Read the model definition and answer for the solid it produces. Units are mm, in the model's axes. A direction names the side the tool comes from. Give positions to 0.01 mm unless a question says otherwise; leave off trailing zeros. Write each loop counter-clockwise with the first axis right and the second up, starting at its lowest first coordinate (ties: lowest second). Pieces come first, ordered by that corner, then holes. Notation, with made-up numbers: (31, 88.5) -> (83, 88.5) arc R20 ccw to (83, 98.5) -> close; hole circle Ø3 at (19, 26). An arc over 180 degrees is marked (long way). Answer as CSV lines item,"result". Start each with the question number.
1. The part is cut by section A-A, the plane y = 27. Determine the outline of the cut face in (x, z), and give its area (4 significant figures).
2. For a pull along X with two mould halves and no side action, classify faces 1 (the cylindrical face through (0.57, 44.14, 4.45)), 2 (the flat face through (-12, -9, 9)), 3 (the cylindrical face through (6.819, 14.377, 4.437)) as pulls with the +X half, pulls with the -X half, needs draft (parallel to the pull), parting line crosses it, or undercut.
3. The part is cut by section B-B, the plane x = 0. Determine the outline of the cut face in (y, z), and give its area (3 significant figures).
4. Given pin 1 (12 mm diameter, centred on x = -27, y = -10.5, fed in from +Z); pin 2 (5 mm diameter, centred on x = 14, z = 7, fed in from +Y); pin 3 (1 mm diameter, centred on x = 6, z = 5, fed in from -Y), each flat-ended and moving along its own axis, determine where each tip first touches the part or whether it passes through.
5. Find the intervals of material crossed by line 1 (Y direction, x = -14.5, z = 2.75); line 2 (X direction, y = -23, z = 5.25); line 3 (Y direction, x = -1, z = 2.75), in increasing order.
6. A tool of negligible diameter and unlimited length cuts with its end or side. For faces 4 (the cylindrical face through (-8.82, -13.48, 4.44)), 5 (the cylindrical face through (-32.866, -20.771, 5.198)), from which of +Z, -Z, +X, -X, +Y, -Y can it reach the whole face along a straight path? Write none if from no direction.
7. The part is cut by section C-C, the plane z = 2.5. Give the number of separate pieces and of enclosed holes in the cut face, and give its area (3 significant figures).
from build123d import *

# Parameters (mm, degrees)
F0_R     = 11.95
F0_R_2   = 1.705642275
F0_R_3   = 11
F1_DEPTH = 9
F2_SIZE  = 1
F0_R_4   = 10
F3_DEPTH = 1.5


# Not quite as in the source:
# - a fillet or chamfer that OpenCascade refuses, or shapes differently, is made with other operations: its cross-section is extruded or revolved along the edge and cut away or added


with BuildPart() as f1:
    # F0 (on Top) → F1 (new body)
    with BuildSketch(Plane.XY):
        with BuildLine():
            ThreePointArc((18.9439392787, 3.0656279209), (11.0053071194, 6.3539170279), (12.1268812973, 14.8731187027))
            ThreePointArc((12.1268812973, 14.8731187027), (0, 44.15), (-12.1268812973, 14.8731187027))
            ThreePointArc((-12.1268812973, 14.8731187027), (-11.0053071194, 6.3539170279), (-18.9439392787, 3.0656279209))
            ThreePointArc((-18.9439392787, 3.0656279209), (-38.2350215771, -22.075), (-6.8170579813, -17.9387466235))
            ThreePointArc((-6.8170579813, -17.9387466235), (0, -12.7078340558), (6.8170579813, -17.9387466235))
            ThreePointArc((6.8170579813, -17.9387466235), (38.2350215771, -22.075), (18.9439392787, 3.0656279209))
        make_face()
        with Locations((-23.3826859022, -13.5)):
            Circle(F0_R, mode=Mode.SUBTRACT)
        with Locations((-7.4659583891, -12.4409667216)):
            Circle(F0_R_2, mode=Mode.SUBTRACT)
        with Locations((-14.5071724231, -0.2452262678)):
            Circle(F0_R_2, mode=Mode.SUBTRACT)
        with Locations((7.4659583891, -12.4409667216)):
            Circle(F0_R_2, mode=Mode.SUBTRACT)
        with Locations((23.3826859022, -13.5)):
            Circle(F0_R, mode=Mode.SUBTRACT)
        Circle(F0_R_3, mode=Mode.SUBTRACT)
        with Locations((14.5071724231, -0.2452262678)):
            Circle(F0_R_2, mode=Mode.SUBTRACT)
        with Locations((-7.041214034, 12.6861929893)):
            Circle(F0_R_2, mode=Mode.SUBTRACT)
        with Locations((7.041214034, 12.6861929893)):
            Circle(F0_R_2, mode=Mode.SUBTRACT)
        with Locations((0, 27)):
            Circle(F0_R, mode=Mode.SUBTRACT)
    extrude(amount=F1_DEPTH)

    # F2
    f2_edges = [f1.edges().sort_by_distance(p)[0] for p in [
        (-38.235022, -22.075, 9),
        (0, -12.707834, 9),
        (38.235022, -22.075, 9),
        (38.235022, -22.075, 0),
        (0, -12.707834, 0),
        (-38.235022, -22.075, 0),
        (-11.005307, 6.353917, 9),
        (-11.005307, 6.353917, 0),
        (0, 44.15, 0),
        (0, 44.15, 9),
        (11.005307, 6.353917, 9),
        (11.005307, 6.353917, 0),
    ]]
    chamfer(f2_edges, length=F2_SIZE)

    # F0 (on Top) → F3 (join)
    with BuildSketch(Plane.XY):
        with Locations((0, 27)):
            Circle(F0_R)
        with Locations((0, 27)):
            Circle(F0_R_4, mode=Mode.SUBTRACT)
        with Locations((-23.3826859022, -13.5)):
            Circle(F0_R)
        with Locations((-23.3826859022, -13.5)):
            Circle(F0_R_4, mode=Mode.SUBTRACT)
        with Locations((23.3826859022, -13.5)):
            Circle(F0_R)
        with Locations((23.3826859022, -13.5)):
            Circle(F0_R_4, mode=Mode.SUBTRACT)
    extrude(amount=F3_DEPTH)

    # F4: chamfer of 1 on 1 edges, made by hand

    # F4_s1 → F4_t2 (revolve, cut)
    with BuildSketch(Plane.XZ):
        Polygon((12, 9), (11, 8), (11, 9), align=None)
    revolve(axis=Axis((0, 0, 9), (0, 0, 1)), mode=Mode.SUBTRACT)


solid = f1.part
Results found:
1,outline,"(-17.15, 1) -> (-16.15, 0) -> (-10, 0) -> (-10, 1.5) -> (-11.95, 1.5) -> (-11.95, 9) -> (-16.15, 9) -> (-17.15, 8) -> close; (10, 0) -> (16.15, 0) -> (17.15, 1) -> (17.15, 8) -> (16.15, 9) -> (11.95, 9) -> (11.95, 1.5) -> (10, 1.5) -> close"
1,area,"97.45 mm²"
2,face 1,"parting line crosses it"
2,face 2,"needs draft"
2,face 3,"undercut"
3,outline,"(-12.71, 1) -> (-11.71, 0) -> (-11, 0) -> (-11, 8) -> (-11.85, 8.85) -> (-12.71, 8) -> close; (11, 0) -> (17, 0) -> (17, 1.5) -> (15.05, 1.5) -> (15.05, 9) -> (12, 9) -> (11, 8) -> close; (37, 0) -> (43.15, 0) -> (44.15, 1) -> (44.15, 8) -> (43.15, 9) -> (38.95, 9) -> (38.95, 1.5) -> (37, 1.5) -> close"
3,area,"101 mm²"
4,pin 1,"stops at z = 1.5"
4,pin 2,"stops at y = 39.72"
4,pin 3,"stops at y = -17.02"
5,line 1,"y = -28.17 to -21.49, -5.51 to -1.95, 1.46 to 3.33, 17.84 to 36.16"
5,line 2,"x = -37.66 to -30.63, -16.13 to -9.1, 9.1 to 16.13, 30.63 to 37.66"
5,line 3,"y = -12.78 to -10.95, 10.95 to 15.09, 38.91 to 44.12"
6,face 4,"+Z, -Z"
6,face 5,"+Z"
7,separate pieces,"1"
7,enclosed holes,"10"
7,area,"1,490 mm²"
